The listing builds one solid part. Answer for the finished solid, in the listing's coordinates (mm). Coordinates: 2 decimals unless noted, no trailing zeros. Order: outer loops, then holes, each group sorted by start corner. A loop starts at its lowest first (then second) coordinate and runs counter-clockwise, first axis right, second up. Notation, with made-up numbers: (34, 16) - (43, 16) arc R21 cw to (43, 39) - close; hole circle Ø5 at (-12.75, 58). An arc over 180 degrees is marked (long way). One line per item, written item: value. Start each with the question number.
```python
from build123d import *

# Parameters (mm, degrees)
F0_R     = 2
F1_DEPTH = 1


with BuildPart() as f1:
    # F0 (on Top) → F1 (new body)
    with BuildSketch(Plane.XY):
        with BuildLine():
            ThreePointArc((-28, -4.5), (-27.853553, -4.853553), (-27.5, -5))
            Line((-27.5, -5), (27.5, -5))
            ThreePointArc((27.5, -5), (27.853553, -4.853553), (28, -4.5))
            Line((28, -4.5), (28, 4))
            Line((28, 4), (-28, 4))
            Line((-28, 4), (-28, -4.5))
        make_face()
        with Locations((-24, 0)):
            Circle(F0_R, mode=Mode.SUBTRACT)
        with Locations((24, 0)):
            Circle(F0_R, mode=Mode.SUBTRACT)
    extrude(amount=F1_DEPTH)


solid = f1.part
```
(1) For a pull along Y with two mould halves and no side action, classify faces 1 (the face through (0.4, 4, 0.5)), 2 (the face through (-0.4, -5, 0.5)), 3 (the face through (22.002, 0.088, 0.493)) as pulls with the +Y half, pulls with the -Y half, needs draft (parallel to the pull), parting line crosses it, or undercut.
(2) The part is cut by section B-B on y = 0. Determine the outline of the cut face in (x, z).
(3) Consider probe 1 along Y at (x, z) = (24, 0.75); probe 2 along X at (y, z) = (-1, 0.45); probe 3 along X at (y, z) = (-0.75, 0.65). Determine where each line is inside the solid, lowest interval first.
(4) The part is cut by section C-C on z = 0.3. Determine the outline of the cut face in (x, y), plus the area to 3 significant figures.
(5) The part is cut by section A-A on x = -24. Determine the outline of the cut face in (y, z).
Completed:
1. face 1: pulls with the +Y half
1. face 2: pulls with the -Y half
1. face 3: undercut
2. outline: (-28, 0) - (-26, 0) - (-26, 1) - (-28, 1) - close; (-22, 0) - (22, 0) - (22, 1) - (-22, 1) - close; (26, 0) - (28, 0) - (28, 1) - (26, 1) - close
3. probe 1: y = -5 to -2, 2 to 4
3. probe 2: x = -28 to -25.73, -22.27 to 22.27, 25.73 to 28
3. probe 3: x = -28 to -25.85, -22.15 to 22.15, 25.85 to 28
4. outline: (-28, -4.5) arc R0.5 ccw to (-27.5, -5) - (27.5, -5) arc R0.5 ccw to (28, -4.5) - (28, 4) - (-28, 4) - close; hole circle Ø4 at (-24, 0); hole circle Ø4 at (24, 0)
4. area: 479 mm2
5. outline: (-5, 0) - (-2, 0) - (-2, 1) - (-5, 1) - close; (2, 0) - (4, 0) - (4, 1) - (2, 1) - close
